from build123d import *

# Parameters (mm, degrees)
CROQUIS1_R              = 15.5
SALIENTE_EXTRUIR1_DEPTH = 65.4
CROQUIS2_R              = 6
SALIENTE_EXTRUIR2_DEPTH = 2
CROQUIS3_R              = 18.3
SALIENTE_EXTRUIR3_DEPTH = 22
CROQUIS4_R              = 1.5
CORTAR_EXTRUIR1_DEPTH   = 20
CROQUIS5_R              = 1.25
CORTAR_EXTRUIR2_DEPTH   = 20
CROQUIS6_R              = 6
SALIENTE_EXTRUIR4_DEPTH = 6
CROQUIS7_R              = 3
SALIENTE_EXTRUIR5_DEPTH = 15


with BuildPart() as part:
    # Croquis1 → Saliente-Extruir1 (new body)
    with BuildSketch(Plane.XY):
        Circle(CROQUIS1_R)
    extrude(amount=SALIENTE_EXTRUIR1_DEPTH)

    # Croquis2 → Saliente-Extruir2 (add)
    with BuildSketch(Plane(origin=(0, 0, 0), x_dir=(-1, 0, 0), z_dir=(0, 0, -1))):
        Circle(CROQUIS2_R)
    extrude(amount=SALIENTE_EXTRUIR2_DEPTH)

    # Croquis3 → Saliente-Extruir3 (add)
    with BuildSketch(Plane.XY.offset(65.4)):
        Circle(CROQUIS3_R)
    extrude(amount=SALIENTE_EXTRUIR3_DEPTH)

    # Croquis4 → Cortar-Extruir1 (cut)
    with BuildSketch(Plane.XY.offset(87.4)):
        with Locations((-15.43, 0)):
            Circle(CROQUIS4_R)
        with Locations((-7.715, 13.36277198)):
            Circle(CROQUIS4_R)
        with Locations((7.715, 13.36277198)):
            Circle(CROQUIS4_R)
        with Locations((15.43, 0)):
            Circle(CROQUIS4_R)
        with Locations((-7.715, -13.36277198)):
            Circle(CROQUIS4_R)
        with Locations((7.715, -13.36277198)):
            Circle(CROQUIS4_R)
    extrude(amount=-CORTAR_EXTRUIR1_DEPTH, mode=Mode.SUBTRACT)

    # Croquis5 → Cortar-Extruir2 (cut)
    with BuildSketch(Plane.XY.offset(87.4)):
        with Locations((0, -15.43)):
            Circle(CROQUIS5_R)
        with Locations((-13.36277198, 7.715)):
            Circle(CROQUIS5_R)
        with Locations((13.36277198, 7.715)):
            Circle(CROQUIS5_R)
    extrude(amount=-CORTAR_EXTRUIR2_DEPTH, mode=Mode.SUBTRACT)

    # Croquis6 → Saliente-Extruir4 (add)
    with BuildSketch(Plane.XY.offset(87.4)):
        with Locations((0, 7.37)):
            Circle(CROQUIS6_R)
    extrude(amount=SALIENTE_EXTRUIR4_DEPTH)

    # Croquis7 → Saliente-Extruir5 (add)
    with BuildSketch(Plane.XY.offset(93.4)):
        with Locations((0, 7.37)):
            Circle(CROQUIS7_R)
    extrude(amount=SALIENTE_EXTRUIR5_DEPTH)


solid = part.part
The model under review builds one solid part; all positions refer to its coordinate system, in mm. A direction names the side the tool comes from. Coordinates: 2 decimals unless noted, no trailing zeros. Loops run counter-clockwise (first coordinate to the right, second up) from the corner with the lowest first, then second, coordinate; pieces in that order, holes last. Notation, with made-up numbers: (41.5, -5) -> (45.5, -5) arc R19 ccw to (45.5, 4) -> close; hole circle Ø8 at (-26, 29). An arc over 180 degrees is marked (long way). Use a Markdown table: item, result. Add a question column.
1. Draft analysis for pull direction Y (two halves, no side actions). For faces 3 (the face through (9.84, 15.43, 76.25)), 4 (the face through (13, 8, 67.4)), 5 (the face through (-8.04, 11.9, 77.54)), 6 (the face through (-14, 8, 65.4)), state which applies: pulls with the +Y half, pulls with the -Y half, needs draft (parallel to the pull), parting line crosses it, or undercut.
2. Machinability: for faces 1 (the face through (-13, 8, 67.4)), 2 (the face through (0, 0, -2)), which of the approach directions +Z, -Z, +X, -X, +Y, -Y give a long, thin tool a straight path to every point of the face, cutting with its end or side? Answer none if there is none.
3. Clearance check with flat-ended pins moving along their axes: pin 1 Ø0.8 at (x, y) = (0.5, -15) entering from +Z; pin 2 Ø1 at (x, z) = (-8.5, 43) entering from +Y; pin 3 Ø4 at (x, y) = (-15.43, 0) entering from -Z. State where each tip first meets the part, or that it passes through.
4. Add section C-C on y = 0. Write out the cut boundary in (x, z).
5. Add section A-A on z = 78. Give the number of separate pieces and of enclosed holes in the cut face, plus the area to 3 significant figures.
6. To check wall thickness, follow line 1 (Y direction, x = 0, z = 78.5); line 2 (Z direction, x = -15, y = 7); line 3 (Y direction, x = -10, z = 37). State the ranges of each line that lie inside material, in increasing order.
7. Add section D-D on z = 13. Write out the cut boundary in (x, y), plus the area to 3 significant figures.
8. Add section B-B on x = 0. Write out the cut boundary in (y, z).
Returned:
| question | item | result |
|---|---|---|
| 1 | face 3 | parting line crosses it |
| 1 | face 4 | undercut |
| 1 | face 5 | undercut |
| 1 | face 6 | needs draft |
| 2 | face 1 | +Z |
| 2 | face 2 | -Z, +X, -X, +Y, -Y |
| 3 | pin 1 | stops at z = 67.4 |
| 3 | pin 2 | stops at y = 13.28 |
| 3 | pin 3 | stops at z = 0 |
| 4 | outline | (-18.3, 65.4) -> (-15.5, 65.4) -> (-15.5, 0) -> (-6, 0) -> (-6, -2) -> (6, -2) -> (6, 0) -> (15.5, 0) -> (15.5, 65.4) -> (18.3, 65.4) -> (18.3, 87.4) -> (16.93, 87.4) -> (16.93, 67.4) -> (13.93, 67.4) -> (13.93, 87.4) -> (-13.93, 87.4) -> (-13.93, 67.4) -> (-16.93, 67.4) -> (-16.93, 87.4) -> (-18.3, 87.4) -> close |
| 5 | separate pieces | 1 |
| 5 | enclosed holes | 9 |
| 5 | area | 995 mm² |
| 6 | line 1 | y = -18.3 to -16.68, -14.18 to 18.3 |
| 6 | line 2 | z = 65.4 to 87.4 |
| 6 | line 3 | y = -11.84 to 11.84 |
| 7 | outline | circle Ø31 at (0, 0) |
| 7 | area | 755 mm² |
| 8 | outline | (-18.3, 65.4) -> (-15.5, 65.4) -> (-15.5, 0) -> (-6, 0) -> (-6, -2) -> (6, -2) -> (6, 0) -> (15.5, 0) -> (15.5, 65.4) -> (18.3, 65.4) -> (18.3, 87.4) -> (13.37, 87.4) -> (13.37, 93.4) -> (10.37, 93.4) -> (10.37, 108.4) -> (4.37, 108.4) -> (4.37, 93.4) -> (1.37, 93.4) -> (1.37, 87.4) -> (-14.18, 87.4) -> (-14.18, 67.4) -> (-16.68, 67.4) -> (-16.68, 87.4) -> (-18.3, 87.4) -> close |
